Here's how the part is built. I have some questions about the finished solid (model axes, mm). Give positions to 0.01 mm unless a question says otherwise; leave off trailing zeros. Loops run counter-clockwise (first coordinate to the right, second up) from the corner with the lowest first, then second, coordinate; pieces in that order, holes last. Notation, with made-up numbers: (-8, 84) -> (51, 84) arc R27 cw to (51, 121) -> close; hole circle Ø6 at (-38.5, -2). An arc over 180 degrees is marked (long way). Answer in a Markdown table with one row per item. Add a question column.
Item 1: If we section it at B-B (y = 10.75): Write out the boundary of the cut face in (x, z).
Item 2: For P1, Ø12, axis at y = 10.5, z = 512, coming from the +X side; P2, Ø11, axis at x = 10.5, z = 351, coming from the +Y side; P3, Ø1.5, axis at y = 9, z = 672, coming from the +X side, each with a flat end and sliding along its axis, tell me the tip position at first contact or that it passes through.
Item 3: If we section it at A-A (z = 316): Write out the boundary of the cut face in (x, y), then the cut area to 3 significant figures.
Item 4: If I drill on line 1 (Y direction, x = 14.5, z = 732.5); line 2 (X direction, y = 4, z = 159.5), over which ranges is the centre line in solid material (lowest first)?
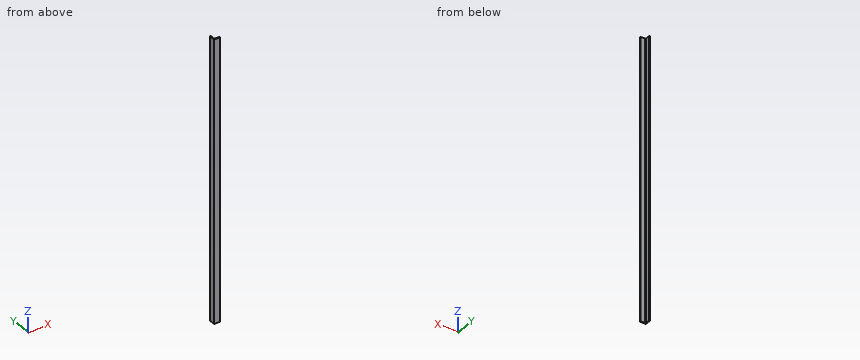
```python
from build123d import *

# Parameters (mm, degrees)
BOSS_EXTRU_1_DEPTH = 955


with BuildPart() as part:
    # Esquisse1 → Boss.-Extru.1 (new body)
    with BuildSketch(Plane.XY):
        with BuildLine():
            Line((0, 0), (0, 20))
            Line((0, 20), (3, 20))
            Line((3, 20), (3, 6))
            ThreePointArc((3, 6), (3.878679656, 3.878679656), (6, 3))
            Line((6, 3), (20, 3))
            Line((20, 3), (20, 0))
            Line((20, 0), (0, 0))
        make_face()
    extrude(amount=BOSS_EXTRU_1_DEPTH)


solid = part.part
```
Recorded:
| question | item | result |
|---|---|---|
| 1 | outline | (0, 0) -> (3, 0) -> (3, 955) -> (0, 955) -> close |
| 2 | P1 | stops at x = 3.4 |
| 2 | P2 | stops at y = 3.17 |
| 2 | P3 | stops at x = 3 |
| 3 | outline | (0, 0) -> (20, 0) -> (20, 3) -> (6, 3) arc R3 cw to (3, 6) -> (3, 20) -> (0, 20) -> close |
| 3 | area | 113 mm^2 |
| 4 | line 1 | y = 0 to 3 |
| 4 | line 2 | x = 0 to 3.76 |
